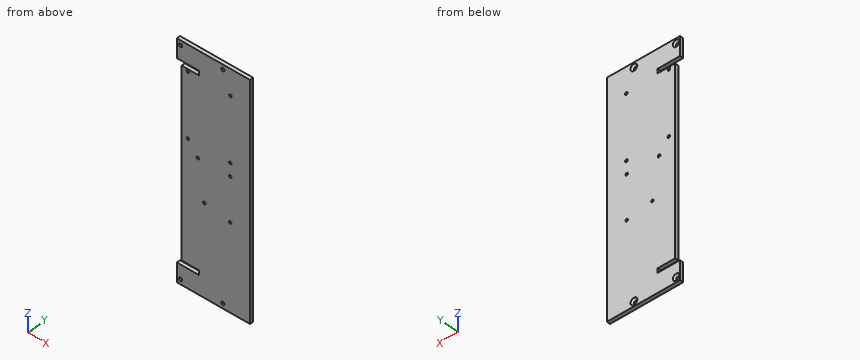
Autodesk Inventor part; units mm, degrees
ref_plane "YZ Plane" through (0, 0, 0) normal (1, 0, 0) x (0, 1, 0)
ref_plane "XZ Plane" through (0, 0, 0) normal (0, 1, 0) x (-1, 0, 0)
ref_plane "XY Plane" through (0, 0, 0) normal (0, 0, 1) x (1, 0, 0)
sketch "Эскиз1" plane through (0, 0, 0) normal (0, 1, 0) x (-1, 0, 0)
  line L0 (-2.6795, -19) -> (83.0251, -19)
  line L1 (-2.6795, 244) -> (83.0251, 244)
  circle A0 centre (30.7479, 238.5) radius 1.85
  circle A1 centre (78.7479, 238.5) radius 1.85
  circle A2 centre (78.7479, -13.5) radius 1.85
  circle A3 centre (30.7479, -13.5) radius 1.85
  line L2 (83.0251, 244) -> (-2.6795, 244)
  line L3 (-2.6795, 244) -> (-2.6795, -19)
  line L4 (-2.6795, -19) -> (83.0251, -19)
  line L5 (83.0251, -19) -> (83.0251, 244)
  point P0 (0, 0)
  point P1 (83.0251, -19)
  point P2 (-2.6795, 244)
  dimension "d7" = 5.5
  dimension "d8" = 5.5
  dimension "d9" = 4.2772
  dimension "d10" = 48
  dimension "d11" = 263
  dimension "d12" = 5.5
  dimension "d13" = 5.5
  dimension "d14" = 4.2772
  dimension "d15" = 48
extrude "Выдавливание1" add sketch "Эскиз1" along normal blind 4
thicken "Толщина1" operation add thickness 2.671 both sides no extend neighbours yes toward (-1, 0, 0) faces at (2.6795, 1.3333, 156.3333)
chamfer "Фаска1" distance 2 angle 45 4 edges at (-76.8979, 4, 238.5) (-28.8979, 4, 238.5) (-28.8979, 4, -13.5) (-76.8979, 4, -13.5)
sketch "Эскиз2" plane through (-1.399, 4, 60) normal (0, 1, 0) x (1, 0, 0)
  line L0 (-76.2625, -157.5) -> (-76.2625, 52.5)
  line L1 (-76.2625, 52.5) -> (-56.2625, 52.5)
  line L2 (-56.2625, -157.5) -> (-76.2625, -157.5)
  line L3 (-56.2625, 57.5) -> (-76.2625, 57.5)
  line L4 (-76.2625, 57.5) -> (-81.2625, 57.5)
  line L5 (-81.2625, 57.5) -> (-81.2625, -162.5)
  line L6 (-81.2625, -162.5) -> (-76.2625, -162.5)
  line L7 (-76.2625, -162.5) -> (-56.2625, -162.5)
  line L8 (-56.2625, -162.5) -> (-56.2625, -157.5)
  line L9 (-56.2625, 52.5) -> (-56.2625, 57.5)
  line L10 (1.4075, -184) -> (1.4075, 79)
  point P0 (0, 0)
  dimension "d21" = 57.67
  dimension "d22" = 25
  dimension "d23" = 5
extrude "Выдавливание2" cut sketch "Эскиз2" against normal blind 10
thicken "Толщина2" operation add thickness 2 both sides no extend neighbours yes toward (-1, 0, 0) faces at (-82.6615, 2.6667, 75.8333)
sketch "Эскиз3" plane through (0, 4, 0) normal (0, 1, 0) x (1, 0, 0)
  circle A0 centre (-51.7551, -83.34) radius 1.5
  circle A1 centre (-22.5451, -78.26) radius 1.5
  circle A2 centre (-22.5451, -127.79) radius 1.5
  circle A3 centre (-59.3751, -127.79) radius 1.5
  circle A4 centre (-22.2251, -142.53) radius 1.5
  circle A5 centre (-70.4851, -142.53) radius 1.5
  circle A6 centre (-22.2251, -214.92) radius 1.5
  circle A7 centre (-70.4851, -214.92) radius 1.5
  point P0 (0, 0)
extrude "Выдавливание3" cut sketch "Эскиз3" against normal blind 10
properties part number "KB33-046-004-002 - Передняя пластина" material "Дерево (вишня)"
Input: part model. Units: mm. Frame: model coordinates. Coordinates: 2 decimals unless noted, no trailing zeros. Write each loop counter-clockwise with the first axis right and the second up, starting at its lowest first coordinate (ties: lowest second). Pieces come first, ordered by that corner, then holes. Notation, with made-up numbers: (40, -27.75) -> (55, -27.75) arc R4 ccw to (55, -23.75) -> close; hole circle Ø2 at (62.5, 88). An arc over 180 degrees is marked (long way). Answer as a JSON object with one key per item and string values.
1. First-contact query: P1, Ø3.5, axis at x = -22.55, z = 78.26, coming from the -Y side; P2, Ø2.5, axis at x = -22.23, z = 142.53, coming from the +Y side; P3, Ø1.2, axis at y = 2.5, z = 5, coming from the -X side. Flat tips, straight axial feed; report the tip coordinate or a pass-through.
Result set:
{"P1": "stops at y = 0", "P2": "passes through", "P3": "stops at x = -57.66"}
2. Section A-A on x = -64. Return the cut outline in (y, z).
Result set:
{"outline": "(0, -19) -> (4, -19) -> (4, 2.5) -> (0, 2.5) -> close; (0, 7.5) -> (4, 7.5) -> (4, 217.5) -> (0, 217.5) -> close; (0, 222.5) -> (4, 222.5) -> (4, 244) -> (0, 244) -> close"}
3. Material intervals for line 1 (Z direction, x = -75.5, y = 3.1); line 2 (X direction, y = 2.1, z = 214.92); line 3 (Z direction, x = -70.5, y = 3.1), sorted ascending. Write a range as from..to.
Result set:
{"line 1": "z = -19..2.5, 7.5..217.5, 222.5..244", "line 2": "x = -77.66..-71.99, -68.99..-23.73, -20.73..0.01", "line 3": "z = -19..2.5, 7.5..141.03, 144.03..213.42, 216.42..217.5, 222.5..244"}
4. Section B-B on z = 38. Return the cut outline in (x, y), then the cut area to 3 significant figures.
Result set:
{"outline": "(-77.66, 0) -> (0.01, 0) -> (0.01, 4) -> (-77.66, 4) -> close", "area": "311 mm2"}
